The model under review builds one solid part; all positions refer to its coordinate system, in mm. A direction names the side the tool comes from. Give positions to 0.01 mm unless a question says otherwise; leave off trailing zeros. Loops run counter-clockwise (first coordinate to the right, second up) from the corner with the lowest first, then second, coordinate; pieces in that order, holes last. Notation, with made-up numbers: (-15.75, -6) - (21.25, -6) arc R14 ccw to (21.25, 9) - close; hole circle Ø4 at (14.5, 42). An arc over 180 degrees is marked (long way). Return JSON: item names as keys, results as strings. Group by question number.
```python
from build123d import *

# Parameters (mm, degrees)
SKETCH1_W           = 200
SKETCH1_H           = 125
BOSS_EXTRUDE1_DEPTH = 70
SKETCH2_W           = 210
SKETCH2_H           = 135
BOSS_EXTRUDE2_DEPTH = 10
SKETCH3_R           = 10
BOSS_EXTRUDE5_DEPTH = 5
CUT_EXTRUDE2_DEPTH  = 5
CUT_EXTRUDE3_DEPTH  = 10
SKETCH10_W          = 10
SKETCH10_H          = 125
CUT_EXTRUDE4_DEPTH  = 10
BOSS_EXTRUDE6_DEPTH = 5
SKETCH12_R          = 8
CUT_EXTRUDE5_DEPTH  = 10
SKETCH15_R          = 4.5
CUT_EXTRUDE6_DEPTH  = 10
SKETCH18_W          = 115
SKETCH18_H          = 2.5
CUT_EXTRUDE7_DEPTH  = 220


with BuildPart() as part:
    # Sketch1 → Boss-Extrude1 (new body)
    with BuildSketch(Plane(origin=(0, 0, 0), x_dir=(1, 0, 0), z_dir=(0, 1, 0))):
        Polygon((210, 0), (0, 0), (0, -135), (5, -135), (210, -135), align=None)
        with Locations((105, -67.5)):
            Rectangle(SKETCH1_W, SKETCH1_H, mode=Mode.SUBTRACT)
    extrude(amount=BOSS_EXTRUDE1_DEPTH)

    # Sketch2 → Boss-Extrude2 (add)
    with BuildSketch(Plane(origin=(0, 0, 0), x_dir=(-1, 0, 0), z_dir=(0, -1, 0))):
        with Locations((-105, -67.5)):
            Rectangle(SKETCH2_W, SKETCH2_H)
    extrude(amount=BOSS_EXTRUDE2_DEPTH)

    # Sketch3 → Boss-Extrude5 (add)
    with BuildSketch(Plane(origin=(0, -10, 0), x_dir=(-1, 0, 0), z_dir=(0, -1, 0))):
        with Locations((-210, 0)):
            Circle(SKETCH3_R)
        Circle(SKETCH3_R)
        with Locations((0, -135)):
            Circle(SKETCH3_R)
        with Locations((-210, -135)):
            Circle(SKETCH3_R)
    extrude(amount=-BOSS_EXTRUDE5_DEPTH)

    # Sketch7 → Cut-Extrude2 (cut)
    with BuildSketch(Plane(origin=(0, -5, 0), x_dir=(1, 0, 0), z_dir=(0, 1, 0))):
        with BuildLine():
            ThreePointArc((215.235533906, -138.535533906), (214.186095741, -136.964938701), (212.333452378, -137.333452378))
            Line((212.333452378, -137.333452378), (214.737615434, -139.737615434))
            ThreePointArc((214.737615434, -139.737615434), (215.106129111, -139.186095741), (215.235533906, -138.535533906))
        make_face()
        with BuildLine():
            Line((214.737615434, -139.737615434), (212.333452378, -137.333452378))
            ThreePointArc((212.333452378, -137.333452378), (212.333452378, -139.737615434), (214.737615434, -139.737615434))
        make_face()
        with BuildLine():
            ThreePointArc((214.737615434, 4.737615434), (212.333452378, 4.737615434), (212.333452378, 2.333452378))
            Line((212.333452378, 2.333452378), (214.737615434, 4.737615434))
        make_face()
        with BuildLine():
            Line((214.737615434, 4.737615434), (212.333452378, 2.333452378))
            ThreePointArc((212.333452378, 2.333452378), (214.186095741, 1.964938701), (215.235533906, 3.535533906))
            ThreePointArc((215.235533906, 3.535533906), (215.106129111, 4.186095741), (214.737615434, 4.737615434))
        make_face()
        with BuildLine():
            ThreePointArc((-4.737615434, 4.737615434), (-4.737615434, 2.333452378), (-2.333452378, 2.333452378))
            Line((-2.333452378, 2.333452378), (-4.737615434, 4.737615434))
        make_face()
        with BuildLine():
            Line((-4.737615434, 4.737615434), (-2.333452378, 2.333452378))
            ThreePointArc((-2.333452378, 2.333452378), (-1.964938701, 2.884972071), (-1.835533906, 3.535533906))
            ThreePointArc((-1.835533906, 3.535533906), (-2.884972071, 5.106129111), (-4.737615434, 4.737615434))
        make_face()
        with BuildLine():
            ThreePointArc((-1.835533906, -138.535533906), (-1.964938701, -137.884972071), (-2.333452378, -137.333452378))
            Line((-2.333452378, -137.333452378), (-4.737615434, -139.737615434))
            ThreePointArc((-4.737615434, -139.737615434), (-2.884972071, -140.106129111), (-1.835533906, -138.535533906))
        make_face()
        with BuildLine():
            Line((-4.737615434, -139.737615434), (-2.333452378, -137.333452378))
            ThreePointArc((-2.333452378, -137.333452378), (-4.737615434, -137.333452378), (-4.737615434, -139.737615434))
        make_face()
    extrude(amount=-CUT_EXTRUDE2_DEPTH, mode=Mode.SUBTRACT)

    # Sketch9 → Cut-Extrude3 (cut)
    with BuildSketch(Plane(origin=(0, 0, 0), x_dir=(1, 0, 0), z_dir=(0, 1, 0))):
        Polygon((195, -130), (200, -125), (205, -120), (205, -15), (200, -10), (195, -5), align=None)
    extrude(amount=-CUT_EXTRUDE3_DEPTH, mode=Mode.SUBTRACT)

    # Sketch10 → Cut-Extrude4 (cut)
    with BuildSketch(Plane(origin=(0, 0, 0), x_dir=(1, 0, 0), z_dir=(0, 1, 0))):
        with Locations((190, -67.5)):
            Rectangle(SKETCH10_W, SKETCH10_H)
    extrude(amount=-CUT_EXTRUDE4_DEPTH, mode=Mode.SUBTRACT)

    # Sketch11 → Boss-Extrude6 (add)
    with BuildSketch(Plane(origin=(0, 70, 0), x_dir=(1, 0, 0), z_dir=(0, 1, 0))):
        with BuildLine():
            ThreePointArc((213.3, -67.5), (215, -65.8), (216.7, -67.5))
            Line((216.7, -67.5), (220, -67.5))
            ThreePointArc((220, -67.5), (217.071067812, -60.428932188), (210, -57.5))
            Line((210, -57.5), (210, -67.5))
            Line((210, -67.5), (213.3, -67.5))
        make_face()
        with BuildLine():
            Line((220, -67.5), (216.7, -67.5))
            ThreePointArc((216.7, -67.5), (215, -69.2), (213.3, -67.5))
            Line((213.3, -67.5), (210, -67.5))
            Line((210, -67.5), (210, -77.5))
            ThreePointArc((210, -77.5), (217.071067812, -74.571067812), (220, -67.5))
        make_face()
        with BuildLine():
            Line((205, -76.160254038), (205, -58.839745962))
            ThreePointArc((205, -58.839745962), (200, -67.5), (205, -76.160254038))
        make_face()
        with BuildLine():
            Line((210, -67.5), (210, -57.5))
            ThreePointArc((210, -57.5), (207.411809549, -57.840741737), (205, -58.839745962))
            Line((205, -58.839745962), (205, -76.160254038))
            ThreePointArc((205, -76.160254038), (207.411809549, -77.159258263), (210, -77.5))
            Line((210, -77.5), (210, -67.5))
        make_face()
        with BuildLine():
            ThreePointArc((10, -67.5), (8.660254038, -62.5), (5, -58.839745962))
            Line((5, -58.839745962), (5, -76.160254038))
            ThreePointArc((5, -76.160254038), (8.660254038, -72.5), (10, -67.5))
        make_face()
        with BuildLine():
            Line((0, -57.5), (0, -67.5))
            Line((0, -67.5), (0, -77.5))
            ThreePointArc((0, -77.5), (2.588190451, -77.159258263), (5, -76.160254038))
            Line((5, -76.160254038), (5, -58.839745962))
            ThreePointArc((5, -58.839745962), (2.588190451, -57.840741737), (0, -57.5))
        make_face()
        with BuildLine():
            Line((0, -77.5), (0, -67.5))
            Line((0, -67.5), (-3.3, -67.5))
            ThreePointArc((-3.3, -67.5), (-5, -69.2), (-6.7, -67.5))
            Line((-6.7, -67.5), (-10, -67.5))
            ThreePointArc((-10, -67.5), (-7.071067812, -74.571067812), (0, -77.5))
        make_face()
        with BuildLine():
            Line((-3.3, -67.5), (0, -67.5))
            Line((0, -67.5), (0, -57.5))
            ThreePointArc((0, -57.5), (-7.071067812, -60.428932188), (-10, -67.5))
            Line((-10, -67.5), (-6.7, -67.5))
            ThreePointArc((-6.7, -67.5), (-5, -65.8), (-3.3, -67.5))
        make_face()
    extrude(amount=-BOSS_EXTRUDE6_DEPTH)

    # Sketch12 → Cut-Extrude5 (cut)
    with BuildSketch(Plane(origin=(0, 0, 0), x_dir=(-1, 0, 0), z_dir=(0, 0, -1))):
        with Locations((-75, 17.5)):
            Circle(SKETCH12_R)
        with Locations((-120, 20)):
            Circle(SKETCH12_R)
    extrude(amount=-CUT_EXTRUDE5_DEPTH, mode=Mode.SUBTRACT)

    # Sketch15 → Cut-Extrude6 (cut)
    with BuildSketch(Plane.XY.offset(135)):
        with Locations((105, 20)):
            Circle(SKETCH15_R)
    extrude(amount=-CUT_EXTRUDE6_DEPTH, mode=Mode.SUBTRACT)

    # Sketch18 → Cut-Extrude7 (cut)
    with BuildSketch(Plane(origin=(210, 0, 0), x_dir=(0, 0, -1), z_dir=(1, 0, 0))):
        with Locations((-67.5, 43.75)):
            Rectangle(SKETCH18_W, SKETCH18_H)
        with Locations((-67.5, 53.75)):
            Rectangle(SKETCH18_W, SKETCH18_H)
        with Locations((-67.5, 33.75)):
            Rectangle(SKETCH18_W, SKETCH18_H)
        with Locations((-67.5, 23.75)):
            Rectangle(SKETCH18_W, SKETCH18_H)
        with Locations((-67.5, 13.75)):
            Rectangle(SKETCH18_W, SKETCH18_H)
    extrude(amount=-CUT_EXTRUDE7_DEPTH, mode=Mode.SUBTRACT)


solid = part.part
```
1) To check wall thickness, follow line 1 (X direction, y = 66.55, z = 67.5); line 2 (Z direction, x = 7.5, y = 4); line 3 (X direction, y = 22, z = 96.5). State the ranges of each line that lie inside material, in increasing order.
2) Draft analysis for pull direction Y (two halves, no side actions). For faces 1 (the face through (-7.3, -7.535, -6.834)), 2 (the face through (208, 55, 68)), 3 (the face through (201, 0, 9)), state which applies: +Y half, -Y half, draft (parallel to the pull), parting line (faces both ways), or undercut.
3) We need section C-C, the plane x = 75. Write out the cut boundary in (y, z), plus the area to 3 significant figures.
4) Tool access review of faces 4 (the face through (200, -5, 125)), 5 (the face through (3, 45, 68)), 6 (the face through (104, 39, 5)), 7 (the face through (203, 65, 67)): name each direction out of +Z, -Z, +X, -X, +Y, -Y from which nothing blocks a thin tool from reaching the whole face with its end or side.
5) We need section B-B, the plane z = 98.5. Count the separate pieces of the cut face and the enclosed holes in it, plus the area to 4 significant figures.
6) For pin 1 Ø3 at (x, y) = (207.5, 54) entering from +Z; pin 2 Ø2 at (x, z) = (53.5, 82) entering from +Y; pin 3 Ø7 at (x, y) = (105, 20) entering from -Z, all flat-tipped, find the tip position at first contact; note any pin that passes through.
7) We need section A-A, the plane x = 105. Write out the cut boundary in (y, z).
Findings:
{
 "1": {"line 1": "x = -10 to -6.7, -3.3 to 10, 200 to 213.3, 216.7 to 220", "line 2": "z = 0 to 5, 130 to 135", "line 3": "x = 0 to 5, 205 to 210"},
 "2": {"face 1": "draft", "face 2": "undercut", "face 3": "+Y half"},
 "3": {"outline": "(-10, 0) - (9.5, 0) - (9.5, 5) - (0, 5) - (0, 130) - (70, 130) - (70, 135) - (-10, 135) - close; (25.5, 0) - (70, 0) - (70, 5) - (25.5, 5) - close", "area": "1,970 mm^2"},
 "4": {"face 4": "+Y, -Y", "face 5": "+X, -X", "face 6": "+Y", "face 7": "-Y"},
 "5": {"separate pieces": "12", "enclosed holes": "0", "area": "2,475 mm^2"},
 "6": {"pin 1": "stops at z = 135", "pin 2": "stops at y = 0", "pin 3": "stops at z = 0"},
 "7": {"outline": "(-10, 0) - (70, 0) - (70, 5) - (0, 5) - (0, 130) - (15.5, 130) - (15.5, 135) - (-10, 135) - close; (24.5, 130) - (70, 130) - (70, 135) - (24.5, 135) - close"}
}
